Read the model definition and answer for the solid it produces. Units are mm, in the model's axes. A direction names the side the tool comes from. Coordinates: 2 decimals unless noted, no trailing zeros. Loops run counter-clockwise (first coordinate to the right, second up) from the corner with the lowest first, then second, coordinate; pieces in that order, holes last.
from build123d import *

# Parameters (mm, degrees)
P_IDAT_VYSUNUT_M1_DEPTH = 3


with BuildPart() as part:
    # Skica1 → Přidat vysunutím1 (new body)
    with BuildSketch(Plane.XY):
        Polygon((20, 3), (23.5, 3), (40, 3), (40, 0), (60, 0), (60, 3), (75, 3), (75, 0), (85, 0), (85, 3), (100, 3), (100, 0), (120, 0), (120, 3), (136.5, 3), (140, 3), (140, 0), (160, 0), (160, 62), (140, 62), (140, 59), (120, 59), (120, 62), (100, 62), (100, 59), (85, 59), (85, 62), (75, 62), (75, 59), (60, 59), (60, 62), (40, 62), (40, 59), (20, 59), (20, 62), (0, 62), (0, 0), (20, 0), align=None)
        Polygon((80, 51.06787282), (62.620712338, 41.03393641), (62.620712338, 20.96606359), (80, 10.93212718), (97.379287662, 20.96606359), (97.379287662, 41.03393641), align=None, mode=Mode.SUBTRACT)
    extrude(amount=P_IDAT_VYSUNUT_M1_DEPTH)


solid = part.part
Item 1: A cutting plane is placed at B-B on x = 66.5. Determine the outline of the cut face in (y, z), then the cut area to 3 significant figures.
Numbers:
outline: (3, 0) - (18.73, 0) - (18.73, 3) - (3, 3) - close; (43.27, 0) - (59, 0) - (59, 3) - (43.27, 3) - close
area: 94.4 mm2
Item 2: Determine the mould class of faces 4 (the face through (130, 59, 1)), 5 (the face through (62.621, 31, 1)), 6 (the face through (71.19, 16.02, 1.48)), 7 (the face through (50, 0, 1)) for opening direction Y: released by +Y, released by -Y, zero draft, split by the parting line, or undercut.
Numbers:
face 4: released by +Y
face 5: undercut
face 6: undercut
face 7: released by -Y
Item 3: Given pin 1 (1.5 mm diameter, centred on x = 93.5, z = 1.5, fed in from -Y); pin 2 (1.5 mm diameter, centred on x = 25.5, z = 2, fed in from +Y); pin 3 (1.5 mm diameter, centred on y = 35.5, z = 1.5, fed in from -X), each flat-ended and moving along its own axis, determine where each tip first touches the part or whether it passes through.
Numbers:
pin 1: stops at y = 3
pin 2: stops at y = 59
pin 3: stops at x = 0
Item 4: A cutting plane is placed at C-C on x = 137. Determine the outline of the cut face in (y, z).
Numbers:
outline: (3, 0) - (59, 0) - (59, 3) - (3, 3) - close
Item 5: Find the intervals of material crossed by line 1 along X through (y, z) = (31.5, 1.05); line 2 along Y through (x, z) = (83, 0.7); line 3 along Y through (x, z) = (25, 0.35), in increasing order.
Numbers:
line 1: x = 0 to 62.62, 97.38 to 160
line 2: y = 0 to 12.66, 49.34 to 62
line 3: y = 3 to 59
Item 6: A cutting plane is placed at A-A on y = 27.5. Determine the outline of the cut face in (x, z).
Numbers:
outline: (0, 0) - (62.62, 0) - (62.62, 3) - (0, 3) - close; (97.38, 0) - (160, 0) - (160, 3) - (97.38, 3) - close
Item 7: Which of the six approach directions +Z, -Z, +X, -X, +Y, -Y give full straight-line access (tool end or side, diameter ignored) to faces 1 (the face through (20, 60, 1)), 2 (the face through (150, 0, 1)), 3 (the face through (75, 2, 1))?
Numbers:
face 1: +Z, -Z, +Y
face 2: +Z, -Z, +X, -X, -Y
face 3: +Z, -Z, -Y
